Here's how the part is built. I have some questions about the finished solid (model axes, mm). A direction names the side the tool comes from. Coordinates: 2 decimals unless noted, no trailing zeros. Write each loop counter-clockwise with the first axis right and the second up, starting at its lowest first coordinate (ties: lowest second). Pieces come first, ordered by that corner, then holes. Notation, with made-up numbers: (-28, 39) -> (5, 39) arc R29 ccw to (5, 77) -> close; hole circle Ø2 at (69.25, 6.5). An arc over 180 degrees is marked (long way). Put each result on its own line as item: value.
```python
from build123d import *

# Parameters (mm, degrees)
EXTRUDE_1_DEPTH     = 3
SKETCH_2_R          = 1.65
CUT_EXTRUDE_1_DEPTH = 3
FILLET_1_R          = 5
CUT_EXTRUDE_2_DEPTH = 0.5


with BuildPart() as part:
    # ｽｹｯﾁ1 → ﾎﾞｽ - 押し出し1 (new body)
    with BuildSketch(Plane.XY):
        Polygon((173.531323483, 340.900859956), (144.605881047, 375.372859896), (133.1152144, 365.731045751), (119.019825089, 370.861347901), (103.628918639, 328.575179965), (117.724307951, 323.444877815), (162.040656836, 331.259045811), align=None)
        Polygon((144.605881047, 375.372859896), (133.1152144, 365.731045751), (119.019825089, 370.861347901), align=None)
    extrude(amount=EXTRUDE_1_DEPTH)

    # ｽｹｯﾁ2 → ｶｯﾄ - 押し出し1 (cut)
    with BuildSketch(Plane.XY.offset(3)):
        with Locations((113.24176437, 333.057723546)):
            Circle(SKETCH_2_R)
        with Locations((123.50236867, 361.24850217)):
            Circle(SKETCH_2_R)
        with Locations((143.681454796, 364.8066195)):
            Circle(SKETCH_2_R)
        with Locations((162.965083087, 341.825286207)):
            Circle(SKETCH_2_R)
    extrude(amount=-CUT_EXTRUDE_1_DEPTH, mode=Mode.SUBTRACT)

    # ﾌｨﾚｯﾄ1
    fillet_1_edges = [part.edges().sort_by_distance(p)[0] for p in [
        (173.531323483, 340.900859956, 1.5),
        (162.040656836, 331.259045811, 1.5),
        (117.724307951, 323.444877815, 1.5),
        (103.628918639, 328.575179965, 1.5),
        (119.019825089, 370.861347901, 1.5),
        (144.605881047, 375.372859896, 1.5),
    ]]
    fillet(fillet_1_edges, radius=FILLET_1_R)

    # ｽｹｯﾁ3 → ｶｯﾄ - 押し出し2 (cut)
    with BuildSketch(Plane.XY.offset(3)):
        Polygon((121.413966092, 377.439196246), (103.628918639, 328.575179965), (117.771292582, 323.427776808), (133.132579218, 365.632564976), (162.002354614, 331.22690643), (173.531323483, 340.900859956), (140.106367779, 380.735170998), (131.711632891, 373.691152049), align=None)
    extrude(amount=-CUT_EXTRUDE_2_DEPTH, mode=Mode.SUBTRACT)


solid = part.part
```
Item 1: Imagine slicing it at C-C on z = 1.85. Write out the boundary of the cut face in (x, y), then the cut area to 3 significant figures.
Output:
outline: (105.34, 333.27) arc R5 ccw to (108.33, 326.87) -> (116.47, 323.9) arc R5 ccw to (119.04, 323.68) -> (160.72, 331.03) arc R5 ccw to (163.07, 332.12) -> (169.7, 337.69) arc R5 ccw to (170.32, 344.73) -> (146.46, 373.16) arc R5 ccw to (141.76, 374.87) -> (121.86, 371.36) arc R5 ccw to (118.03, 368.15) -> close; hole circle Ø3.3 at (113.24, 333.06); hole circle Ø3.3 at (123.5, 361.25); hole circle Ø3.3 at (143.68, 364.81); hole circle Ø3.3 at (162.97, 341.83)
area: 2,280 mm²
Item 2: Please list where these lines run through material, in increasing order: line 1 along Z through (x, y) = (125.5, 354); line 2 along Y through (x, z) = (162, 0.3); line 3 along X through (y, z) = (332, 2.05). Write a range as from..to.
Output:
line 1: z = 0..2.5
line 2: y = 331.43..340.49, 343.16..354.64
line 3: x = 105.06..111.98, 114.51..162.92
Item 3: Imagine slicing it at B-B on y = 339. Write out the boundary of the cut face in (x, z), then the cut area to 3 significant figures.
Output:
outline: (107.42, 0) -> (170.81, 0) -> (170.81, 2.5) -> (155.48, 2.5) -> (155.48, 3) -> (123.44, 3) -> (123.44, 2.5) -> (107.42, 2.5) -> close
area: 174 mm²
Item 4: Imagine slicing it at D-D on x = 156.5. Write out the boundary of the cut face in (y, z).
Output:
outline: (330.28, 0) -> (361.2, 0) -> (361.2, 2.5) -> (337.78, 2.5) -> (337.78, 3) -> (330.28, 3) -> close
Item 5: If we mould it in two halves opening along Y, with no side actions, what happens to faces 4 (the flat face through (166.338, 334.865, 1.232)), 5 (the flat face through (138, 361, 2.5)), 6 (the cylindrical face through (112.884, 331.447, 1.268)), 7 (the flat face through (111.775, 350.955, 1.232))? For each: released by +Y, released by -Y, zero draft, split by the parting line, or undercut.
Output:
face 4: released by -Y
face 5: zero draft
face 6: undercut
face 7: released by +Y
Item 6: Which directions (+Z, -Z, +X, -X, +Y, -Y) give clear straight access to the entire face, cutting with the end or side of a thin tool? Please do faces 1 (the flat face through (147.303, 348.745, 2.754)), 2 (the cylindrical face through (145.255, 365.302, 1.268)), 3 (the flat face through (125.38, 344.33, 2.75)).
Output:
face 1: +Z, +X, +Y
face 2: +Z, -Z
face 3: +Z, -X, +Y
Item 7: Imagine slicing it at A-A on x = 112.5. Write out the boundary of the cut face in (y, z), then the cut area to 3 significant figures.
Output:
outline: (325.35, 0) -> (331.58, 0) -> (331.58, 2.5) -> (325.35, 2.5) -> close; (334.53, 0) -> (352.95, 0) -> (352.95, 2.5) -> (334.53, 2.5) -> close
area: 61.6 mm²
Item 8: For P1, Ø1, axis at y = 336.5, z = 2.5, coming from the -X side; P2, Ø5.5, axis at x = 162.97, y = 341.83, coming from the -Z side; P3, Ø5.5, axis at x = 113.24, y = 333.06, coming from the +Z side, each with a flat end and sliding along its axis, tell me the tip position at first contact or that it passes through.
Output:
P1: stops at x = 106.33
P2: stops at z = 0
P3: stops at z = 2.5
